from build123d import *

# Parameters (mm, degrees)
SKIZZE1_R                       = 70
SKIZZE1_R_2                     = 15.75
AUFSATZ_LINEAR_AUSTRAGEN1_DEPTH = 20
SKIZZE2_W                       = 2
SKIZZE2_H                       = 44.25


with BuildPart() as part:
    # Skizze1 → Aufsatz-Linear austragen1 (new body)
    with BuildSketch(Plane.XY):
        Circle(SKIZZE1_R)
        Circle(SKIZZE1_R_2, mode=Mode.SUBTRACT)
    extrude(amount=AUFSATZ_LINEAR_AUSTRAGEN1_DEPTH)

    # Skizze2 → Schnitt-Rotation1 (revolve, cut)
    with BuildSketch(Plane(origin=(0, 0, 0), x_dir=(0, 0, -1), z_dir=(1, 0, 0)), mode=Mode.PRIVATE) as schnitt_rotation1_sk:
        with Locations((-19, 42.875)):
            Rectangle(SKIZZE2_W, SKIZZE2_H)
        with Locations((-1, 42.875)):
            Rectangle(SKIZZE2_W, SKIZZE2_H)
    revolve(schnitt_rotation1_sk.sketch.rotate(Axis((0, 0, 0), (0, 0, 1)), 90), axis=Axis((0, 0, 0), (0, 0, 1)), mode=Mode.SUBTRACT)


solid = part.part
Geometry: final body of the model. Coordinates: model frame, mm. A direction names the side the tool comes from. Give positions to 0.01 mm unless a question says otherwise; leave off trailing zeros. Order: outer loops, then holes, each group sorted by start corner. A loop starts at its lowest first (then second) coordinate and runs counter-clockwise, first axis right, second up. Notation, with made-up numbers: (38.5, -37.75) - (52.5, -37.75) arc R17 ccw to (52.5, -10.75) - close; hole circle Ø11 at (-12.5, 42). An arc over 180 degrees is marked (long way). Use CSV: the item, a comma, the result in double quotes.
1. Mould query, pull axis Z, two halves, no side actions, for faces 4 (the face through (-19.8, -6.2, 19)), 5 (the face through (-15, -15, 2)), 6 (the face through (20.4, -61.9, 20)). Classes: +Z half, -Z half, draft (parallel to the pull), parting line (faces both ways), or undercut.
Answers below:
face 4,"draft"
face 5,"-Z half"
face 6,"+Z half"
2. Section query A-A (y = 0). Output: boundary loops of the cut face in (x, z).
Answers below:
outline,"(-70, 0) - (-65, 0) - (-65, 2) - (-20.75, 2) - (-20.75, 0) - (-15.75, 0) - (-15.75, 20) - (-20.75, 20) - (-20.75, 18) - (-65, 18) - (-65, 20) - (-70, 20) - close; (15.75, 0) - (20.75, 0) - (20.75, 2) - (65, 2) - (65, 0) - (70, 0) - (70, 20) - (65, 20) - (65, 18) - (20.75, 18) - (20.75, 20) - (15.75, 20) - close"
3. Contact query for flat-ended pins moving along their axis: pin 1 (12 mm diameter, centred on y = 41.5, z = 14.5, fed in from -X); pin 2 (12 mm diameter, centred on x = 30, y = 14.5, fed in from +Z); pin 3 (1.5 mm diameter, centred on y = 31.5, z = 16, fed in from -X); pin 4 (1.5 mm diameter, centred on x = 1.5, y = 14.5, fed in from +Z). Output: stop coordinate, or through.
Answers below:
pin 1,"x = -60.33"
pin 2,"z = 18"
pin 3,"x = -62.88"
pin 4,"through"
4. Access query for faces 1 (the face through (-55.55, -42.594, 9.86)), 2 (the face through (-62, -19.52, 0.99)), 3 (the face through (-62, -19.52, 18.99)). Directions: +Z, -Z, +X, -X, +Y, -Y. A direction counts if a zero-diameter tool reaches every point of the face in a straight line with its end or side. Return the directions, or none.
Answers below:
face 1,"+Z, -Z"
face 2,"-Z"
face 3,"+Z"
5. Section query C-C (z = 12). Output: boundary loops of the cut face in (x, y).
Answers below:
outline,"circle Ø140 at (0, 0); hole circle Ø31.5 at (0, 0)"
6. Material intervals for line 1 along Y through (x, z) = (0, 0.85); line 2 along Z through (x, y) = (-29, 56.5); line 3 along X through (y, z) = (43.5, 1.5), sorted ascending. Write a range as from..to.
Answers below:
line 1,"-70..-65, -20.75..-15.75, 15.75..20.75, 65..70"
line 2,"2..18"
line 3,"-54.84..-48.3, 48.3..54.84"
7. Section query D-D (x = -43). Output: boundary loops of the cut face in (y, z).
Answers below:
outline,"(-55.24, 0) - (-48.74, 0) - (-48.74, 2) - (48.74, 2) - (48.74, 0) - (55.24, 0) - (55.24, 20) - (48.74, 20) - (48.74, 18) - (-48.74, 18) - (-48.74, 20) - (-55.24, 20) - close"
